Autodesk Inventor part; units mm, degrees
ref_plane "YZ Plane" through (0, 0, 0) normal (1, 0, 0) x (0, 1, 0)
ref_plane "XZ Plane" through (0, 0, 0) normal (0, 1, 0) x (-1, 0, 0)
ref_plane "XY Plane" through (0, 0, 0) normal (0, 0, 1) x (1, 0, 0)
sketch "Sketch1" plane through (0, 0, 0) normal (0, 0, 1) x (1, 0, 0)
  line L0 (0, 0) -> (50.8, 0)
  line L1 (0, 0) -> (0, 50.8)
  line L2 (0, 50.8) -> (19.05, 50.8)
  arc A0 (101.9948, 132.2372) -> (19.05, 110.0122) centre (63.5, 110.0122) ccw
  arc A1 (85.497, 122.7122) -> (38.1, 110.0122) centre (63.5, 110.0122) ccw
  line L3 (85.497, 122.7122) -> (101.9948, 132.2372)
  line L4 (19.05, 110.0122) -> (19.05, 50.8)
  line L5 (38.1, 110.0122) -> (38.1, 63.5)
  arc A2 (50.8, 25.4) -> (50.8, 50.8) centre (50.8, 38.1) ccw
  arc A3 (38.1, 63.5) -> (50.8, 50.8) centre (50.8, 63.5) ccw
  line L6 (50.8, 0) -> (50.8, 25.4)
  dimension "d5" = 25.4
  dimension "d6" = 44.45
  dimension "d38" = 50.8
  dimension "d65" = 30
  dimension "d84" = 12.7
  dimension "d85" = 12.7
  dimension "d89" = 73.025
  dimension "d90" = 19.05
  dimension "d99" = 0
  dimension "d123" = 50.8
  dimension "d124" = 25.4
extrude "Extrusion1" add sketch "Sketch1" along normal blind 9.525
sketch "Sketch11" plane through (0, 0, 9.525) normal (0, 0, 1) x (1, 0, 0)
  line L0 (0, 0) -> (50.8, 0)
  arc A0 (50.8, 25.4) -> (50.8, 50.8) centre (50.8, 38.1) ccw
  arc A1 (38.1, 63.5) -> (50.8, 50.8) centre (50.8, 63.5) ccw
  line L1 (38.1, 63.5) -> (38.1, 110.0122)
  arc A2 (85.497, 122.7122) -> (38.1, 110.0122) centre (63.5, 110.0122) ccw
  line L2 (85.497, 122.7122) -> (101.9948, 132.2372)
  arc A3 (101.9948, 132.2372) -> (19.05, 110.0122) centre (63.5, 110.0122) ccw
  line L3 (19.05, 110.0122) -> (19.05, 50.8)
  line L4 (19.05, 50.8) -> (0, 50.8)
  line L5 (0, 50.8) -> (0, 0)
  line L6 (50.8, 0) -> (50.8, 25.4)
hole "Hole3" at (50.8, 38.1, 9.525) direction (0, 0, -1) diameter 6.35 end through all
sketch "Sketch12" plane through (0, 50.8, 0) normal (0, 1, 0) x (1, 0, 0)
  line L0 (19.05, 0) -> (0, 0)
  line L1 (0, 0) -> (0, -9.525)
  line L2 (19.05, -9.525) -> (0, -9.525)
  line L3 (19.05, 0) -> (19.05, -9.525)
  point P0 (9.525, -4.7625)
  dimension "d108" = 4.7625
  dimension "d109" = 4.7625
  dimension "d110" = 9.525
sketch "Sketch14" plane through (50.8, 0, 0) normal (1, 0, 0) x (0, 0, -1)
  line L0 (0, 0) -> (0, 25.4)
  line L1 (0, 25.4) -> (-9.525, 25.4)
  line L2 (-9.525, 0) -> (-9.525, 25.4)
  line L3 (0, 0) -> (-9.525, 0)
  point P0 (-4.7625, 9.525)
  dimension "d125" = 4.7625
  dimension "d126" = 4.7625
  dimension "d127" = 9.525
hole "Hole5" at (50.8, 9.525, 4.7625) direction (-0.7071, 0.7071, 0) diameter 5.5626 end through all both
fillet "Fillet7" radius 3.175 5 edges at (50.8, 0, 4.7625) (0, 0, 4.7625) (0, 50.8, 4.7625) (85.497, 122.7122, 4.7625) (101.9948, 132.2372, 4.7625)
sketch "Sketch15" plane through (0, 0, 9.525) normal (0, 0, 1) x (1, 0, 0)
  arc A0 (99.1393, 130.5885) -> (100.1712, 135.1325) centre (97.5518, 133.3382) ccw
  arc A1 (100.1712, 135.1325) -> (19.05, 110.0122) centre (63.5, 110.0122) ccw
  line L0 (19.05, 110.0122) -> (19.05, 50.8)
  line L1 (19.05, 50.8) -> (3.175, 50.8)
  arc A2 (3.175, 50.8) -> (0, 47.625) centre (3.175, 47.625) ccw
  line L2 (0, 47.625) -> (0, 3.175)
  arc A3 (0, 3.175) -> (3.175, 0) centre (3.175, 3.175) ccw
  line L3 (3.175, 0) -> (47.625, 0)
  arc A4 (47.625, 0) -> (50.8, 3.175) centre (47.625, 3.175) ccw
  line L4 (50.8, 3.175) -> (50.8, 25.4)
  arc A5 (50.8, 25.4) -> (50.8, 50.8) centre (50.8, 38.1) ccw
  arc A6 (38.1, 63.5) -> (50.8, 50.8) centre (50.8, 63.5) ccw
  line L5 (38.1, 63.5) -> (38.1, 110.0122)
  arc A7 (83.9497, 125.0777) -> (38.1, 110.0122) centre (63.5, 110.0122) ccw
  arc A8 (83.9497, 125.0777) -> (88.0934, 124.2112) centre (86.5059, 126.9608) ccw
  line L6 (88.0934, 124.2112) -> (99.1393, 130.5885)
  circle A9 centre (50.8, 38.1) radius 3.175
  line L7 (-3.175, 3.175) -> (-3.175, 47.625)
  arc A10 (3.175, 53.975) -> (-3.175, 47.625) centre (3.175, 47.625) ccw
  line L8 (3.175, 53.975) -> (15.875, 53.975)
  line L9 (15.875, 53.975) -> (15.875, 110.0122)
  arc A11 (102.7905, 136.9268) -> (15.875, 110.0122) centre (63.5, 110.0122) ccw
  arc A12 (100.7268, 127.8389) -> (102.7905, 136.9268) centre (97.5518, 133.3382) ccw
  line L10 (100.7268, 127.8389) -> (89.6809, 121.4616)
  arc A13 (81.3935, 123.1945) -> (89.6809, 121.4616) centre (86.5059, 126.9608) ccw
  arc A14 (81.3935, 123.1945) -> (41.275, 110.0122) centre (63.5, 110.0122) ccw
  line L11 (41.275, 110.0122) -> (41.275, 63.5)
  arc A15 (41.275, 63.5) -> (50.8, 53.975) centre (50.8, 63.5) ccw
  arc A16 (53.975, 22.5457) -> (50.8, 53.975) centre (50.8, 38.1) ccw
  line L12 (53.975, 22.5457) -> (53.975, 3.175)
  arc A17 (47.625, -3.175) -> (53.975, 3.175) centre (47.625, 3.175) ccw
  line L13 (47.625, -3.175) -> (3.175, -3.175)
  arc A18 (-3.175, 3.175) -> (3.175, -3.175) centre (3.175, 3.175) ccw
  point P0 (0, 0)
  dimension "d138" = 3.175
properties part number "CLB_041_ScissorHook"
Check sheet for the modelled part. Datum: model origin and axes. Units: mm. A direction names the side the tool comes from. Round coordinates to 2 decimals unless told otherwise and drop trailing zeros. Loops run counter-clockwise (first coordinate to the right, second up) from the corner with the lowest first, then second, coordinate; pieces in that order, holes last.
1. Mould release check, pull along Y, two halves, no side actions. Record for faces 5 (the cylindrical face through (0.95, 49.89, 4.83)), 6 (the flat face through (35, 60, 9.525)), 7 (the cylindrical face through (55.15, 134, 4.7)): released by +Y, released by -Y, zero draft, split by the parting line, or undercut.
2. Scan lines: probe 1 along Y at (x, z) = (45, 4.5); probe 2 along X at (y, z) = (38.1, 2.75) (3 decimals); probe 3 along Y at (x, z) = (48.5, 3.75). Record each from-to range of solid material in increasing order.
3. Sectioned sample at D-D on x = 94. Record the boundary of the cut face in (y, z) (3 decimals).
4. Gauge pin test, flat ends, axial feed: pin 1 Ø3 at (x, z) = (8.5, 3.5) entering from +Y; pin 2 Ø1 at (y, z) = (50, 2.5) entering from -X; pin 3 Ø10 at (x, y) = (50.8, 38.1) entering from -Z; pin 4 Ø3 at (y, z) = (128, 7.5) entering from -X. Record the tip position at first contact, or that the pin passes through.
5. Sectioned sample at C-C on y = 95.5. Record the boundary of the cut face in (x, z) (3 decimals).
6. Sectioned sample at A-A on z = 5.5. Give the number of separate pieces and of enclosed holes in the cut face, and give its area (3 significant figures).
7. Set-up check for faces 1 (the flat face through (38.1, 87, 5)), 2 (the flat face through (50.8, 14, 5)), 3 (the flat face through (19.05, 81, 5)), 4 (the flat face through (0, 25, 5)): record each of +Z, -Z, +X, -X, +Y, -Y from which the full face is reachable in a straight line by a thin tool's end or side.
Recorded:
1. face 5: released by +Y
1. face 6: zero draft
1. face 7: undercut
2. probe 1: y = 0 to 11.41, 19.24 to 52.2, 127.42 to 150.43
2. probe 2: x = 0 to 19.51, 24.94 to 47.625, 53.975 to 63.5
2. probe 3: y = 0.12 to 8.16, 15.49 to 35.91, 40.29 to 51.01, 130.51 to 151.85
3. outline: (127.621, 0) - (142.347, 0) - (142.347, 9.525) - (127.621, 9.525) - close
4. pin 1: stops at y = 50.8
4. pin 2: stops at x = 0.61
4. pin 3: stops at z = 0
4. pin 4: stops at x = 22.22
5. outline: (19.05, 0) - (38.1, 0) - (38.1, 9.525) - (19.05, 9.525) - close
6. separate pieces: 2
6. enclosed holes: 1
6. area: 5,380 mm2
7. face 1: +Z, -Z, +X
7. face 2: +Z, -Z, +X, -Y
7. face 3: +Z, -Z, -X, +Y
7. face 4: +Z, -Z, -X, +Y, -Y
